Part model, mm, in its own coordinate system. A direction names the side the tool comes from. Coordinates: 2 decimals unless noted, no trailing zeros. Order: outer loops, then holes, each group sorted by start corner. A loop starts at its lowest first (then second) coordinate and runs counter-clockwise, first axis right, second up. Notation, with made-up numbers: M 53,30 L 82,30 A16 cw 82,60 Z; hole C -29.5,5.5 d6. An arc over 180 degrees is marked long. Write item = value, one per line. Start each with the question number.
from build123d import *

# Parameters (mm, degrees)
SKETCH3_W           = 5
SKETCH3_H           = 40
BOSS_EXTRUDE1_DEPTH = 4.7752


with BuildPart() as part:
    # Sketch3 → Boss-Extrude1 (new body)
    with BuildSketch(Plane.XY):
        with Locations((-2.5, 20)):
            Rectangle(SKETCH3_W, SKETCH3_H)
        with BuildLine():
            Line((0, 5), (0, 0))
            ThreePointArc((0, 0), (20, 20), (0, 40))
            Line((0, 40), (0, 35))
            ThreePointArc((0, 35), (15, 20), (0, 5))
        make_face()
    extrude(amount=BOSS_EXTRUDE1_DEPTH)


solid = part.part
Item 1: Wall check: line 1 along X through (y, z) = (20.5, 1.1); line 2 along Y through (x, z) = (7.75, 0.5); line 3 along Y through (x, z) = (10.5, 1). Give the ranges that are in metal, low to high. Write a range as [from, to].
Item 2: 3-axis set-ups, long thin cutter, end or side, ignore diameter. For faces 1 (the flat face through (-3, 0, 2)), 2 (the flat face through (0, 20, 2)): which of +Z, -Z, +X, -X, +Y, -Y reach the whole face in a straight line?
Item 3: Cut at C-C, the plane x = 11.5. Write the cut outline in (y, z), and give its area (3 significant figures).
Item 4: Cut at D-D, the plane y = 36. Write the cut outline in (x, z).
Item 5: Flat gauge pins, fed straight in: pin 1 (1 mm diameter, centred on x = 9.5, z = 1.5, fed in from +Y); pin 2 (2.5 mm diameter, centred on y = 21, z = 2.5, fed in from +X); pin 3 (1.5 mm diameter, centred on y = 30, z = 4, fed in from +X). Where does each tip first touch, or does it go through?
Item 6: Cut at A-A, the plane z = 0.95. Write the cut outline in (x, y), and give its area (3 significant figures).
Item 7: Cut at B-B, the plane y = 20. Write the cut outline in (x, z).
Filled sheet:
q1.line_1 = [-5, 0], [14.99, 19.99]
q1.line_2 = [1.56, 7.16], [32.84, 38.44]
q1.line_3 = [2.98, 9.29], [30.71, 37.02]
q2.face_1 = +Z, -Z, +X, -X, -Y
q2.face_2 = +Z, -Z
q3.outline = M 3.64,0 L 10.37,0 L 10.37,4.78 L 3.64,4.78 Z; M 29.63,0 L 36.36,0 L 36.36,4.78 L 29.63,4.78 Z
q3.area = 64.3 mm2
q4.outline = M -5,0 L 12,0 L 12,4.78 L -5,4.78 Z
q5.pin_1 = 37.86
q5.pin_2 = 20
q5.pin_3 = 17.73
q6.outline = M -5,0 L 0,0 A20 ccw 0,40 L -5,40 Z; hole M 0,5 A15 ccw 0,35 Z
q6.area = 475 mm2
q7.outline = M -5,0 L 0,0 L 0,4.78 L -5,4.78 Z; M 15,0 L 20,0 L 20,4.78 L 15,4.78 Z
